Verification items for the finished model (mm, model axes). A direction names the side the tool comes from. Round coordinates to 2 decimals unless told otherwise and drop trailing zeros. Loops run counter-clockwise (first coordinate to the right, second up) from the corner with the lowest first, then second, coordinate; pieces in that order, holes last. Notation, with made-up numbers: M 63.25,71.25 L 88.25,71.25 A35 cw 88.25,103.25 Z; hole C -10.75,-7.5 d3. An arc over 180 degrees is marked long. Write item = value, one per line. Start each with the question number.
from build123d import *

# Parameters (mm, degrees)
SKETCH1_R           = 3.5
BOSS_EXTRUDE1_DEPTH = 12


with BuildPart() as part:
    # Sketch1 → Boss-Extrude1 (new body)
    # profile 1 of 5: a face of its own
    with BuildSketch(Plane(origin=(0, 0, 0), x_dir=(0, 1, 0), z_dir=(0, 0, 1))):
        Polygon((10, -3), (10, -7), (7, -10), (3, -10), (0, -7), (0, -3), (3, 0), (7, 0), align=None)
        with Locations((5, -5)):
            Circle(SKETCH1_R, mode=Mode.SUBTRACT)
    # profile 2 of 5: a face of its own
    with BuildSketch(Plane(origin=(0, 0, 0), x_dir=(0, 1, 0), z_dir=(0, 0, 1))):
        with BuildLine():
            ThreePointArc((7.872281323, -3), (5, -1.5), (2.127718677, -3))
            Line((2.127718677, -3), (7.872281323, -3))
        make_face()
    # profile 3 of 5: a face of its own
    with BuildSketch(Plane(origin=(0, 0, 0), x_dir=(0, 1, 0), z_dir=(0, 0, 1))):
        with BuildLine():
            Line((7.872281323, -7), (2.127718677, -7))
            ThreePointArc((2.127718677, -7), (5, -8.5), (7.872281323, -7))
        make_face()
    # profile 4 of 5: a face of its own
    with BuildSketch(Plane(origin=(0, 0, 0), x_dir=(0, 1, 0), z_dir=(0, 0, 1))):
        with BuildLine():
            Line((2, -6.802775638), (2, -3.197224362))
            ThreePointArc((2, -3.197224362), (1.5, -5), (2, -6.802775638))
        make_face()
    # profile 5 of 5: a face of its own
    with BuildSketch(Plane(origin=(0, 0, 0), x_dir=(0, 1, 0), z_dir=(0, 0, 1))):
        with BuildLine():
            ThreePointArc((8.5, -5), (8.372684391, -4.064585653), (8, -3.197224362))
            Line((8, -3.197224362), (8, -6.802775638))
            ThreePointArc((8, -6.802775638), (8.372684391, -5.935414347), (8.5, -5))
        make_face()
    extrude(amount=BOSS_EXTRUDE1_DEPTH)


solid = part.part
1. Section check D-D, the plane x = 9.75. Enter the section's corners in (y, z), and give its area (3 significant figures).
2. Thickness scan on line 1 (Y direction, x = 4.5, z = 9.75); line 2 (X direction, y = 3.5, z = 9.75); line 3 (Y direction, x = 1, z = 9.5). Record the ranges inside material, lowest first.
3. Tool access check on faces 1 (the flat face through (5, 8, 6)), 2 (the flat face through (9, 2, 6)). Record the directions out of +Z, -Z, +X, -X, +Y, -Y that give a thin tool (end or side, any length) a straight path to the whole face; none if there is none.
4. Section check A-A, the plane y = 6.75. Enter the section's corners in (x, z).
5. Mould release check, pull along X, two halves, no side actions. Record for faces 3 (the flat face through (7, 5, 6)), 4 (the flat face through (0, 5, 6)), 5 (the flat face through (10, 5, 6)): pulls with the +X half, pulls with the -X half, needs draft (parallel to the pull), parting line crosses it, or undercut.
6. Section check C-C, the plane x = 6. Enter the section's corners in (y, z).
7. Section check B-B, the plane z = 0.75. Enter the section's corners in (x, y).
Computed values:
q1.outline = M 2.75,0 L 7.25,0 L 7.25,12 L 2.75,12 Z
q1.area = 54.0 mm2
q2.line_1 = 0 to 2, 8 to 10
q2.line_2 = 0 to 3, 7 to 10
q2.line_3 = 2 to 8
q3.face_1 = +Z, -Z
q3.face_2 = +Z, -Z, +X, -Y
q4.outline = M 0,0 L 3,0 L 3,12 L 0,12 Z; M 7,0 L 10,0 L 10,12 L 7,12 Z
q5.face_3 = undercut
q5.face_4 = pulls with the -X half
q5.face_5 = pulls with the +X half
q6.outline = M 0,0 L 2,0 L 2,12 L 0,12 Z; M 8,0 L 10,0 L 10,12 L 8,12 Z
q7.outline = M 0,3 L 3,0 L 7,0 L 10,3 L 10,7 L 7,10 L 3,10 L 0,7 Z; hole M 3,2.13 A3.5 ccw 3.2,2 L 6.8,2 A3.5 ccw 7,2.13 L 7,7.87 A3.5 ccw 6.8,8 L 3.2,8 A3.5 ccw 3,7.87 Z
